from build123d import *

# Parameters (mm, degrees)
SKETCH1_W                      = 15
SKETCH1_H                      = 2
BOSS_EXTRUDE1_DEPTH            = 7
BOSS_EXTRUDE1_2_DEPTH          = 7
SKETCH2_W                      = 15
SKETCH2_H                      = 7
BOSS_EXTRUDE2_DEPTH            = 2
BOSS_EXTRUDE3_DEPTH            = 9
BOSS_EXTRUDE4_DEPTH            = 2
M3_CLEARANCE_HOLE1_D           = 3.2
M3_CLEARANCE_HOLE1_CSINK_D     = 3.45
M3_CLEARANCE_HOLE1_CSINK_ANGLE = 90
M3_CLEARANCE_HOLE2_D           = 3.2
M3_CLEARANCE_HOLE2_CSINK_D     = 3.45
M3_CLEARANCE_HOLE2_CSINK_ANGLE = 90
FILLET2_R                      = 2
FILLET3_R                      = 2


with BuildPart() as part:
    # Sketch1 → Boss-Extrude1 (new body)
    with BuildSketch(Plane.XY):
        with Locations((51, 4)):
            Rectangle(SKETCH1_W, SKETCH1_H)
    extrude(amount=-BOSS_EXTRUDE1_DEPTH)



with BuildPart() as body_2:
    # Sketch1 → Boss-Extrude1 2 (new body)
    with BuildSketch(Plane.XY):
        with Locations((51, -1)):
            Rectangle(SKETCH1_W, SKETCH1_H)
    extrude(amount=-BOSS_EXTRUDE1_2_DEPTH)


with BuildPart() as part_1:
    add(part.part)

    add(body_2.part)  # Boss-Extrude2 merges body 2
    # Sketch2 → Boss-Extrude2 (add)
    with BuildSketch(Plane.XY):
        with Locations((51, 1.5)):
            Rectangle(SKETCH2_W, SKETCH2_H)
    extrude(amount=BOSS_EXTRUDE2_DEPTH)

    # Sketch3 → Boss-Extrude3 (add)
    with BuildSketch(Plane.XY.offset(2)):
        Polygon((49.332085067, -2), (51.907060552, -2), (46.23047622, 5), (43.655500735, 5), align=None)
        Polygon((52.9075543, -6.409039515), (54.460967148, -5.149313939), (51.907060552, -2), (49.332085067, -2), align=None)
        Polygon((50.092939448, 5), (55.76952378, -2), (58.344499265, -2), (52.667914933, 5), align=None)
        Polygon((47.539032852, 8.149313939), (50.092939448, 5), (52.667914933, 5), (49.0924457, 9.409039515), align=None)
        Polygon((43.655500735, 5), (46.23047622, 5), (45.208913582, 6.259725576), align=None)
        Polygon((58.344499265, -2), (55.76952378, -2), (56.791086418, -3.259725576), align=None)
    extrude(amount=BOSS_EXTRUDE3_DEPTH)

    # Sketch4 → Boss-Extrude4 (add)
    with BuildSketch(Plane.XY.offset(2)):
        Polygon((43.655500735, 5), (52.9075543, -6.409039515), (58.344499265, -2), (49.0924457, 9.409039515), align=None)
    extrude(amount=BOSS_EXTRUDE4_DEPTH)

    # M3 Clearance Hole1 (through all)
    with Locations(Plane(origin=(34.219216483, 27.749752594, 0), x_dir=(0, 0, -1), z_dir=(0.7767064235919557, 0.6298627878760529, 0))):
        with Locations((-7.5, -34.802441812), (-7.5, -27.113443281)):
            CounterSinkHole(M3_CLEARANCE_HOLE1_D / 2, M3_CLEARANCE_HOLE1_CSINK_D / 2, counter_sink_angle=M3_CLEARANCE_HOLE1_CSINK_ANGLE)

    # M3 Clearance Hole2 (through all)
    with Locations(Plane(origin=(0, -2, 0), x_dir=(-1, 0, 0), z_dir=(0, -1, 0))):
        with Locations((-47, 3.5), (-55, 3.5)):
            CounterSinkHole(M3_CLEARANCE_HOLE2_D / 2, M3_CLEARANCE_HOLE2_CSINK_D / 2, counter_sink_angle=M3_CLEARANCE_HOLE2_CSINK_ANGLE)

    # Fillet2
    # the kernel refuses this fillet: 2 mm, written as the material it adds along each edge
    with BuildSketch(Plane(origin=(63.344499265, -2, 2), x_dir=(0, -1, 0), z_dir=(-1, 0, 0))) as fillet2_piece_1_section:
        with BuildLine():
            CenterArc((FILLET2_R, -FILLET2_R), FILLET2_R, 90, 90)
            Line((0, -FILLET2_R), (0, 0))
            Line((0, 0), (FILLET2_R, 0))
        make_face()
    fillet2_piece_1 = extrude(amount=19.012414198, mode=Mode.PRIVATE)
    fillet2_piece_1 = split(fillet2_piece_1, bisect_by=Plane(origin=(51.286566394, -4.410141115, 1.532384034), z_dir=(0.776706423591956, 0.6298627878760524, 0)), keep=Keep.TOP, mode=Mode.PRIVATE)
    fillet2_piece_1 = split(fillet2_piece_1, bisect_by=Plane(origin=(55.372467702, -4.410141115, 1.532384034), z_dir=(-0.6298627878760494, 0.7767064235919585, 0)), keep=Keep.TOP, mode=Mode.PRIVATE)
    add(fillet2_piece_1)
    with BuildSketch(Plane(origin=(38.655500735, 5, 2), x_dir=(0, 0, -1), z_dir=(1, 0, 0))) as fillet2_piece_2_section:
        with BuildLine():
            CenterArc((FILLET2_R, FILLET2_R), FILLET2_R, 180, 90)
            Line((0, FILLET2_R), (0, 0))
            Line((0, 0), (FILLET2_R, 0))
        make_face()
    fillet2_piece_2 = extrude(amount=19.012414198, mode=Mode.PRIVATE)
    fillet2_piece_2 = split(fillet2_piece_2, bisect_by=Plane(origin=(46.627532298, 7.410141115, 1.532384034), z_dir=(0.6298627878760538, -0.776706423591955, 0)), keep=Keep.TOP, mode=Mode.PRIVATE)
    fillet2_piece_2 = split(fillet2_piece_2, bisect_by=Plane(origin=(50.713433606, 7.410141115, 1.532384034), z_dir=(-0.776706423591956, -0.6298627878760528, 0)), keep=Keep.TOP, mode=Mode.PRIVATE)
    add(fillet2_piece_2)

    # Fillet3
    # the kernel refuses this fillet: 2 mm, written as the material it adds along each edge
    with BuildSketch(Plane(origin=(52.481399006, -5.883532118, 2), x_dir=(-0.7767064235919561, -0.6298627878760525, 0), z_dir=(-0.6298627878760524, 0.7767064235919561, 0))) as fillet3_piece_1_section:
        with BuildLine():
            CenterArc((FILLET3_R, FILLET3_R), FILLET3_R, 180, 90)
            Line((0, FILLET3_R), (0, 0))
            Line((0, 0), (FILLET3_R, 0))
        make_face()
    fillet3_piece_1 = extrude(amount=19.012414198, mode=Mode.PRIVATE)
    fillet3_piece_1 = split(fillet3_piece_1, bisect_by=Plane(origin=(46.164389013, 5, 2.465360244), z_dir=(0, -1, 0)), keep=Keep.TOP, mode=Mode.PRIVATE)
    fillet3_piece_1 = split(fillet3_piece_1, bisect_by=Plane(origin=(43.5, 1.248668865, 2.465360244), z_dir=(1, 0, 0)), keep=Keep.TOP, mode=Mode.PRIVATE)
    fillet3_piece_1 = split(fillet3_piece_1, bisect_by=Plane(origin=(46.164389013, -2, 2.465360244), z_dir=(0, 1, 0)), keep=Keep.TOP, mode=Mode.PRIVATE)
    add(fillet3_piece_1)
    with BuildSketch(Plane(origin=(61.493813205, -5.883532118, 2), x_dir=(0, 0, 1), z_dir=(-0.6298627878760524, 0.776706423591956, 0))) as fillet3_piece_2_section:
        with BuildLine():
            CenterArc((FILLET3_R, FILLET3_R), FILLET3_R, 180, 90)
            Line((0, FILLET3_R), (0, 0))
            Line((0, 0), (FILLET3_R, 0))
        make_face()
    fillet3_piece_2 = extrude(amount=19.012414198, mode=Mode.PRIVATE)
    fillet3_piece_2 = split(fillet3_piece_2, bisect_by=Plane(origin=(58.444828917, 5, 2.691548942), z_dir=(0, -1, 0)), keep=Keep.TOP, mode=Mode.PRIVATE)
    fillet3_piece_2 = split(fillet3_piece_2, bisect_by=Plane(origin=(58.5, -1.960151195, 2.691548942), z_dir=(-1, 0, 0)), keep=Keep.TOP, mode=Mode.PRIVATE)
    fillet3_piece_2 = split(fillet3_piece_2, bisect_by=Plane(origin=(58.444828917, -2, 2.691548942), z_dir=(0, 1, 0)), keep=Keep.TOP, mode=Mode.PRIVATE)
    add(fillet3_piece_2)


solid = part_1.part
Here's how the part is built. I have some questions about the finished solid (model axes, mm). A direction names the side the tool comes from. Give positions to 0.01 mm unless a question says otherwise; leave off trailing zeros. Order: outer loops, then holes, each group sorted by start corner. A loop starts at its lowest first (then second) coordinate and runs counter-clockwise, first axis right, second up. Notation, with made-up numbers: (86, -19) -> (138, -19) arc R9 ccw to (138, -13) -> close; hole circle Ø11 at (-12.75, 52.25). An arc over 180 degrees is marked (long way). One line per item, written item: value. Start each with the question number.
1. Will these pins go through, and if not, where does the flat tip stop? pin 1 Ø1.5 at (x, y) = (53.5, 2) entering from -Z; pin 2 Ø4 at (x, z) = (47, -3.5) entering from -Y; pin 3 Ø1 at (y, z) = (7.5, 2) entering from -X; pin 4 Ø1.9 at (x, z) = (47, -3.5) entering from -Y.
2. Imagine slicing it at B-B, the plane z = -3.5. List the corners of the cut face in (x, y) for me (3 decimals), plus the area to 3 significant figures.
3. Imagine slicing it at C-C, the plane x = 47. Count the separate pieces of the cut face and the enclosed holes in it, plus the area to 3 significant figures.
4. I need wall thicknesses on probe 1 along Y at (x, z) = (57.5, -0.75); probe 2 along Z at (x, y) = (47, 4.4); probe 3 along Z at (x, y) = (47, 4). Which ranges of each line are inside material? Lowest first, please. Write a range as from..to.
5. For faces 1 (the face through (51, 0, -3)), 2 (the face through (49, 8, 2)), 3 (the face through (53, -5, 2)), 4 (the face through (58, 4, 2)), 5 (the face through (44, -1, 2)), which set-ups out of +Z, -Z, +X, -X, +Y, -Y let a thin tool reach every point of the face, with its end or its side?
6. Imagine slicing it at D-D, the plane y = 8.5. List the corners of the cut face in (x, z) for me.
7. We'd pull the mould along Z, two halves only. Please class faces 6 (the face through (56.29, -1.17, 7.15)), 7 (the face through (51, 2, 0)), 8 (the face through (51, -2, -3)), 9 (the face through (50.42, 6.07, 5.9)): released by +Z, released by -Z, zero draft, split by the parting line, or undercut.
8. Imagine slicing it at A-A, the plane z = -1. List the corners of the cut face in (x, y) for me.
Values follow:
1. pin 1: stops at z = 0
1. pin 2: stops at y = -2
1. pin 3: stops at x = 46.12
1. pin 4: passes through
2. outline: (43.5, -2) -> (45.275, -2) -> (45.4, -1.875) -> (45.4, 0) -> (43.5, 0) -> close; (43.5, 3) -> (45.4, 3) -> (45.4, 5) -> (43.5, 5) -> close; (48.6, -1.875) -> (48.725, -2) -> (53.275, -2) -> (53.4, -1.875) -> (53.4, 0) -> (48.6, 0) -> close; (48.6, 3) -> (53.4, 3) -> (53.4, 5) -> (48.6, 5) -> close; (56.6, -1.875) -> (56.725, -2) -> (58.5, -2) -> (58.5, 0) -> (56.6, 0) -> close; (56.6, 3) -> (58.5, 3) -> (58.5, 5) -> (56.6, 5) -> close
2. area: 34.4 mm2
3. separate pieces: 3
3. enclosed holes: 0
3. area: 59.5 mm2
4. probe 1: y = -2..0, 3..5
4. probe 2: z = -7..-5.1, -1.9..4
4. probe 3: z = -7..-5.1, -1.9..6.02, 8.98..11
5. face 1: -Z, +X, -X
5. face 2: -Z, +X, -X, +Y
5. face 3: -Z, +X, -X, -Y
5. face 4: +Z, +X, +Y
5. face 5: +Z, -X, -Y
6. outline: (47.97, 2) -> (49.83, 2) -> (49.83, 11) -> (47.97, 11) -> close
7. face 6: undercut
7. face 7: released by -Z
7. face 8: zero draft
7. face 9: undercut
8. outline: (43.5, -2) -> (58.5, -2) -> (58.5, 0) -> (43.5, 0) -> close; (43.5, 3) -> (58.5, 3) -> (58.5, 5) -> (43.5, 5) -> close
